from build123d import *

# Parameters (mm, degrees)
SKETCH1_R           = 2.55
BOSS_EXTRUDE1_DEPTH = 5
SKETCH_1_R          = 5
SKETCH_1_R_2        = 15
CUT_EXTRUDE_1_DEPTH = 2


with BuildPart() as part:
    # Sketch1 → Boss-Extrude1 (new body)
    with BuildSketch(Plane(origin=(0, 0, 0), x_dir=(1, 0, 0), z_dir=(0, 1, 0))):
        with BuildLine():
            Line((52, -40), (-52, -40))
            ThreePointArc((-52, -40), (-54.121320344, -39.121320344), (-55, -37))
            Line((-55, -37), (-55, 37))
            ThreePointArc((-55, 37), (-54.121320344, 39.121320344), (-52, 40))
            Line((-52, 40), (52, 40))
            ThreePointArc((52, 40), (54.121320344, 39.121320344), (55, 37))
            Line((55, 37), (55, -37))
            ThreePointArc((55, -37), (54.121320344, -39.121320344), (52, -40))
        make_face()
        with Locations(Location((-30.3, 30, 0), (0, 0, 270))):
            Circle(SKETCH1_R, mode=Mode.SUBTRACT)
        with Locations(Location((0, 10, 0), (0, 0, 270))):
            Circle(SKETCH1_R, mode=Mode.SUBTRACT)
        with Locations(Location((0, 0, 0), (0, 0, 270))):
            Circle(SKETCH1_R, mode=Mode.SUBTRACT)
        with Locations(Location((10, 0, 0), (0, 0, 270))):
            Circle(SKETCH1_R, mode=Mode.SUBTRACT)
        with Locations(Location((-10, 0, 0), (0, 0, 90))):
            Circle(SKETCH1_R, mode=Mode.SUBTRACT)
        with Locations(Location((-45.8, 15.5, 0), (0, 0, 270))):
            Circle(SKETCH1_R, mode=Mode.SUBTRACT)
        with Locations(Location((30.3, 30, 0), (0, 0, 270))):
            Circle(SKETCH1_R, mode=Mode.SUBTRACT)
        with Locations(Location((0, -10, 0), (0, 0, 90))):
            Circle(SKETCH1_R, mode=Mode.SUBTRACT)
        with Locations(Location((-14.8, 15.5, 0), (0, 0, 270))):
            Circle(SKETCH1_R, mode=Mode.SUBTRACT)
        with Locations(Location((14.8, 15.5, 0), (0, 0, 90))):
            Circle(SKETCH1_R, mode=Mode.SUBTRACT)
        with Locations(Location((45.8, 15.5, 0), (0, 0, 90))):
            Circle(SKETCH1_R, mode=Mode.SUBTRACT)
        with Locations(Location((30.3, -30, 0), (0, 0, 90))):
            Circle(SKETCH1_R, mode=Mode.SUBTRACT)
        with Locations(Location((45.8, -15.5, 0), (0, 0, 270))):
            Circle(SKETCH1_R, mode=Mode.SUBTRACT)
        with Locations(Location((14.8, -15.5, 0), (0, 0, 270))):
            Circle(SKETCH1_R, mode=Mode.SUBTRACT)
        with Locations(Location((-14.8, -15.5, 0), (0, 0, 90))):
            Circle(SKETCH1_R, mode=Mode.SUBTRACT)
        with Locations(Location((-45.8, -15.5, 0), (0, 0, 90))):
            Circle(SKETCH1_R, mode=Mode.SUBTRACT)
        with Locations(Location((-30.3, -30, 0), (0, 0, 90))):
            Circle(SKETCH1_R, mode=Mode.SUBTRACT)
    extrude(amount=BOSS_EXTRUDE1_DEPTH)

    # 草圖1 → 除料-伸長1 (cut)
    with BuildSketch(Plane(origin=(0, 5, 0), x_dir=(1, 0, 0), z_dir=(0, 1, 0))):
        with Locations(Location((-30.3, -30, 0), (0, 0, 270))):
            Circle(SKETCH_1_R)
        with Locations(Location((-30.3, 30, 0), (0, 0, 270))):
            Circle(SKETCH_1_R)
        with Locations(Location((30.3, -30, 0), (0, 0, 270))):
            Circle(SKETCH_1_R)
        with Locations(Location((30.3, 30, 0), (0, 0, 270))):
            Circle(SKETCH_1_R)
        with Locations(Location((0, 0, 0), (0, 0, 270))):
            Circle(SKETCH_1_R_2)
    extrude(amount=-CUT_EXTRUDE_1_DEPTH, mode=Mode.SUBTRACT)


solid = part.part
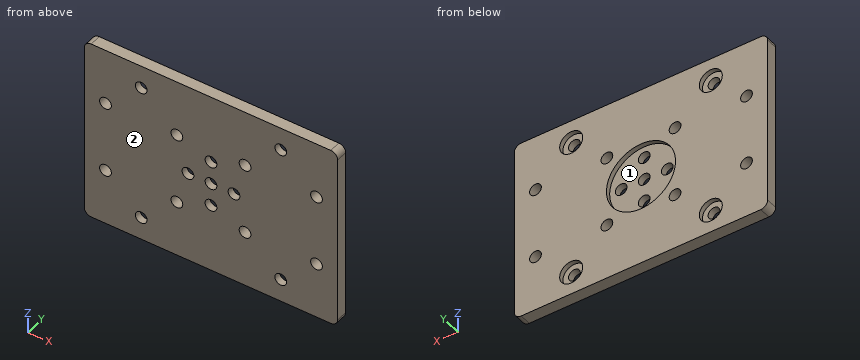
For this review, take the finished solid that the model builds, in its own axes (mm). Face numbers are marked on the shaded views. Coordinates: 2 decimals unless noted, no trailing zeros. Order: outer loops, then holes, each group sorted by start corner. A loop starts at its lowest first (then second) coordinate and runs counter-clockwise, first axis right, second up. Notation, with made-up numbers: (22, -27) -> (62, -27) arc R26 cw to (62, 5) -> close; hole circle Ø10 at (44, -28). An arc over 180 degrees is marked (long way). Return JSON: item names as keys, results as strings.
1. For line 1 (X direction, y = 4.3, z = 30); line 2 (Z direction, x = -30, y = 0.5); line 3 (X direction, y = 2.2, z = 15.5), list the stretches that pass through material, from the lowest coordinate up. Write a range as from..to.
Answer block:
{"line 1": "-55..-35.3, -25.3..25.3, 35.3..55", "line 2": "-40..-32.53, -27.47..27.47, 32.53..40", "line 3": "-55..-48.35, -43.25..-17.35, -12.25..12.25, 17.35..43.25, 48.35..55"}
2. We need section D-D on x = 45.8. Write out the cut boundary in (y, z), and give its area (3 significant figures).
Answer block:
{"outline": "(0, -40) -> (5, -40) -> (5, -18.05) -> (0, -18.05) -> close; (0, -12.95) -> (5, -12.95) -> (5, 12.95) -> (0, 12.95) -> close; (0, 18.05) -> (5, 18.05) -> (5, 40) -> (0, 40) -> close", "area": "349 mm²"}
3. We need section C-C on y = 1.7. State how many separate pieces and enclosed holes the cut face has, and give its area (4 significant figures).
Answer block:
{"separate pieces": "1", "enclosed holes": "17", "area": "8,445 mm²"}
4. We need section A-A on x = 0. Write out the cut boundary in (y, z).
Answer block:
{"outline": "(0, -40) -> (5, -40) -> (5, -15) -> (3, -15) -> (3, -12.55) -> (0, -12.55) -> close; (0, -7.45) -> (3, -7.45) -> (3, -2.55) -> (0, -2.55) -> close; (0, 2.55) -> (3, 2.55) -> (3, 7.45) -> (0, 7.45) -> close; (0, 12.55) -> (3, 12.55) -> (3, 15) -> (5, 15) -> (5, 40) -> (0, 40) -> close"}
5. The part is to be moulded in two halves that separate along X. For the marked faces 1 and 2, say which applies: +X half, -X half, draft (parallel to the pull), parting line (faces both ways), or undercut.
Answer block:
{"face 1": "undercut", "face 2": "draft"}
6. For pin 1 Ø5 at (x, z) = (3.5, 2.5) entering from +Y; pin 2 Ø4 at (x, z) = (-45.8, -15.5) entering from +Y, all flat-tipped, find the tip position at first contact; note any pin that passes through.
Answer block:
{"pin 1": "y = 3", "pin 2": "through"}
7. We need section B-B on z = 30. Write out the cut boundary in (x, y).
Answer block:
{"outline": "(-55, 0) -> (-32.85, 0) -> (-32.85, 3) -> (-35.3, 3) -> (-35.3, 5) -> (-55, 5) -> close; (-27.75, 0) -> (27.75, 0) -> (27.75, 3) -> (25.3, 3) -> (25.3, 5) -> (-25.3, 5) -> (-25.3, 3) -> (-27.75, 3) -> close; (32.85, 0) -> (55, 0) -> (55, 5) -> (35.3, 5) -> (35.3, 3) -> (32.85, 3) -> close"}
